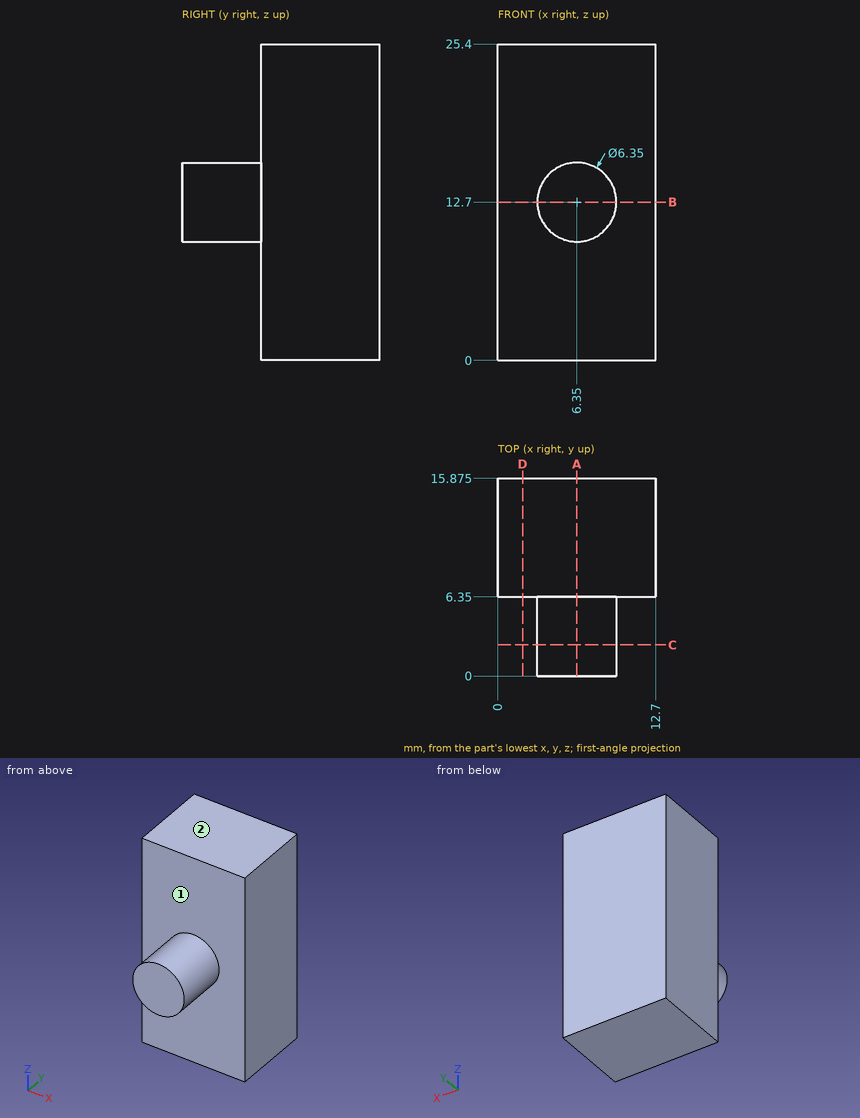
Print and shaded views of the part. All mm, measured from the part's lowest x, y and z. A direction names the side the tool comes from. Coordinates: 2 decimals unless noted, no trailing zeros. Write each loop counter-clockwise with the first axis right and the second up, starting at its lowest first coordinate (ties: lowest second). Pieces come first, ordered by that corner, then holes. Notation, with made-up numbers: (-18.5, 47) -> (39.5, 47) arc R18 ccw to (39.5, 70) -> close; hole circle Ø8 at (29.25, 47.5). An arc over 180 degrees is marked (long way). Use CSV: the item, a comma, the result in double quotes. Start each with the question number.
Q1. Cut at B-B, the plane z = 12.7. List the corners of the cut face in (x, y) (3 decimals), then the cut area to 3 significant figures.
Q2. 3-axis set-ups, long thin cutter, end or side, ignore diameter. For the marked faces 1 and 2: which of +Z, -Z, +X, -X, +Y, -Y reach the whole face in a straight line?
Q3. Cut at C-C, the plane y = 2.5. List the corners of the cut face in (x, z) (3 decimals).
Q4. Cut at D-D, the plane x = 2. List the corners of the cut face in (y, z) (3 decimals), then the cut area to 3 significant figures.
Q5. Cut at A-A, the plane x = 6.35. List the corners of the cut face in (y, z) (3 decimals), then the cut area to 3 significant figures.
Q6. Drill centre lines: probe 1 along Y at (x, z) = (3, 18.75) (3 decimals); probe 2 along Z at (x, y) = (6.5, 6); probe 3 along Z at (x, y) = (6.75, 5.5). Where is each one in solid material? Low to high.
Checked values:
1,outline,"(0, 6.35) -> (3.175, 6.35) -> (3.175, 0) -> (9.525, 0) -> (9.525, 6.35) -> (12.7, 6.35) -> (12.7, 15.875) -> (0, 15.875) -> close"
1,area,"161 mm²"
2,face 1,"-Y"
2,face 2,"+Z, +X, -X, +Y, -Y"
3,outline,"circle Ø6.35 at (6.35, 12.7)"
4,outline,"(6.35, 0) -> (15.875, 0) -> (15.875, 25.4) -> (6.35, 25.4) -> close"
4,area,"242 mm²"
5,outline,"(0, 9.525) -> (6.35, 9.525) -> (6.35, 0) -> (15.875, 0) -> (15.875, 25.4) -> (6.35, 25.4) -> (6.35, 15.875) -> (0, 15.875) -> close"
5,area,"282 mm²"
6,probe 1,"y = 6.35 to 15.875"
6,probe 2,"z = 9.53 to 15.87"
6,probe 3,"z = 9.55 to 15.85"
